Print and shaded views of the part. All mm, measured from the part's lowest x, y and z. Coordinates: 2 decimals unless noted, no trailing zeros. Loops run counter-clockwise (first coordinate to the right, second up) from the corner with the lowest first, then second, coordinate; pieces in that order, holes last. Notation, with made-up numbers: M 34,-36 L 58,-36 A21 cw 58,-16 Z; hole C -13,3.25 d3. An arc over 180 degrees is marked long. Answer as a JSON object with one key per item and string values. Group by question number.
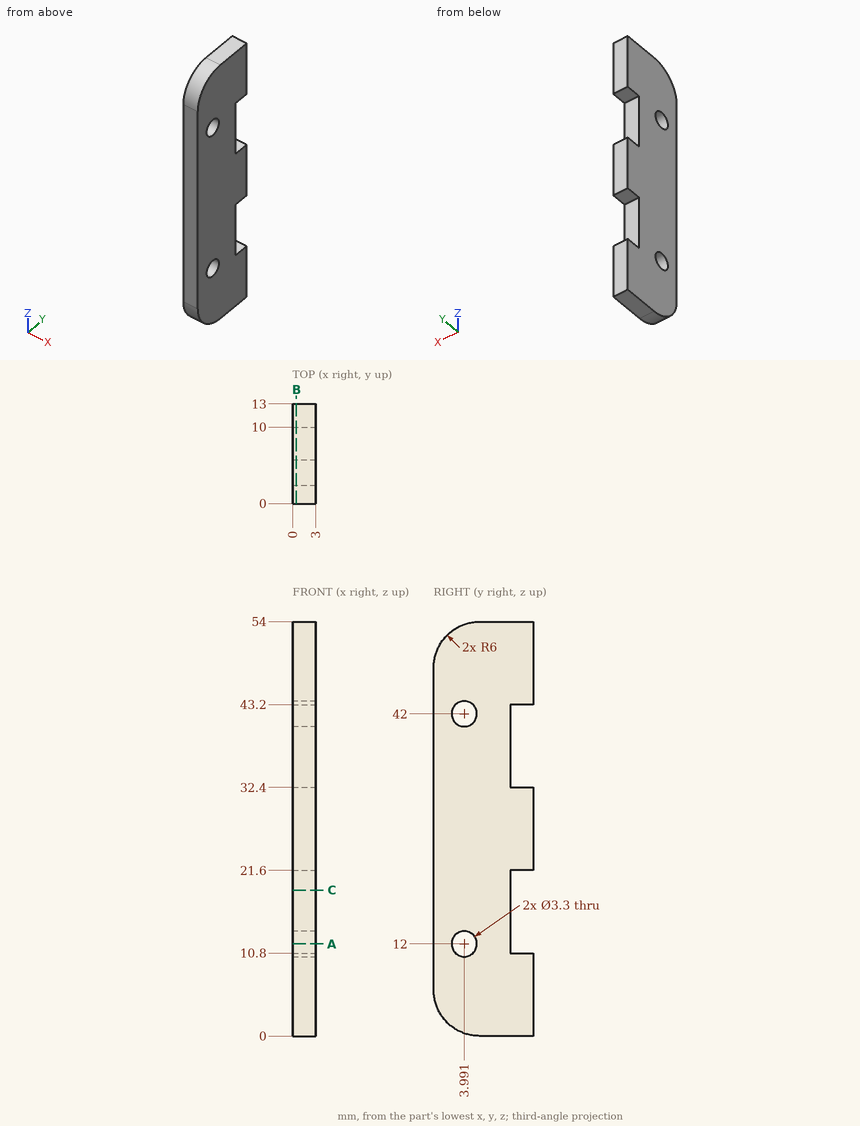
Item 1: Slice it at B-B, the plane x = 0.5. Write the cut outline in (y, z).
Item 2: Pin check, flat tip, straight feed: pin 1 (0.9 mm diameter, centred on x = 2, z = 35.5, fed in from +Y). Stop position of the tip, or through.
Item 3: Slice it at A-A, the plane z = 12. Write the cut outline in (x, y), then the cut area to 3 significant figures.
Item 4: Drill centre lines: L1, parallel to Z at x = 2.55, y = 10.75; L2, parallel to Y at x = 1.5, z = 12; L3, parallel to Z at x = 0.3, y = 2.5. Where is each one in solid material? Low to high. Write a range as from..to.
Item 5: Slice it at C-C, the plane z = 19. Write the cut outline in (x, y), then the cut area to 3 significant figures.
Computed:
{
 "1": {"outline": "M 0,6 A6 ccw 6,0 L 13,0 L 13,10.8 L 10,10.8 L 10,21.6 L 13,21.6 L 13,32.4 L 10,32.4 L 10,43.2 L 13,43.2 L 13,54 L 6,54 A6 ccw 0,48 Z; hole C 3.99,12 d3.3; hole C 3.99,42 d3.3"},
 "2": {"pin 1": "y = 10"},
 "3": {"outline": "M 0,0 L 3,0 L 3,2.34 L 0,2.34 Z; M 0,5.64 L 3,5.64 L 3,10 L 0,10 Z", "area": "20.1 mm2"},
 "4": {"L1": "0..10.8, 21.6..32.4, 43.2..54", "L2": "0..2.34, 5.64..10", "L3": "1.13..11.29, 12.71..41.29, 42.71..52.87"},
 "5": {"outline": "M 0,0 L 3,0 L 3,10 L 0,10 Z", "area": "30.0 mm2"}
}
